For this review, take the finished solid that the model builds, in its own axes (mm). A direction names the side the tool comes from. Coordinates: 2 decimals unless noted, no trailing zeros. Write each loop counter-clockwise with the first axis right and the second up, starting at its lowest first coordinate (ties: lowest second). Pieces come first, ordered by that corner, then holes. Notation, with made-up numbers: (-18, 26) -> (35, 26) arc R21 ccw to (35, 50) -> close; hole circle Ø10 at (-14.5, 58.25). An arc over 180 degrees is marked (long way). One line per item, written item: value. Start each with the question number.
1) Machinability: for faces 1 (the flat face through (16, -6.528, 2)), 2 (the flat face through (124.565, 17.321, 1.478)), 3 (the flat face through (-38.1, -18, 2)), which of the approach directions +Z, -Z, +X, -X, +Y, -Y give a long, thin tool a straight path to every point of the face, cutting with its end or side? Answer none if there is none.
2) Add section D-D (z = 2.2). State how many separate pieces and enclosed holes the cut face has, and give its area (3 significant figures).
3) For probe 1 along Y at (x, z) = (76.2, 1.85); probe 2 along Y at (x, z) = (104.5, 2.55); probe 3 along Y at (x, z) = (127, 1.6), list the stretches that pass through material, from the lowest coordinate up. Write a range as from..to.
4) For pin 1 Ø4 at (x, y) = (76.2, 41.07) entering from -Z; pin 2 Ø0.9 at (y, z) = (-17, 1) entering from +X; pin 3 Ø0.9 at (y, z) = (-17.5, 2) entering from -X; pin 4 Ø0.9 at (x, z) = (30, 1) entering from -Y, all flat-tipped, find the tip position at first contact; note any pin that passes through.
5) Add section C-C (y = 25.4). State the section outline as (x, z) points.
6) Add section A-A (x = 76.2). State the section outline as (y, z) points.
7) Mouldability with a two-part tool opening along X and no side actions: class faces 4 (the flat face through (74.696, 8.434, 1.52)), 5 (the flat face through (70.38, -7.28, 1.48)), 6 (the flat face through (23, 15, 0)) as released by +X, released by -X, zero draft, split by the parting line, or undercut.
8) Add section B-B (x = 127). State the section outline as (y, z) points, and give its area (3 significant figures).
from build123d import *

# Parameters (mm, degrees)
BASE_DEPTH              = 2.9972
JOINT_HOLES_D           = 4.3053
JOINT_HOLES_DEPTH       = 6.351016
OUTER_FILLET_R          = 6.35
SKETCH5_W               = 12.7
SKETCH5_H               = 2.9972
BASE_PLATE_SLOTS_DEPTH  = 142.562822885
UNDER_PLATE_SLOTS_DEPTH = 142.562822885
TOP_PLATE_SLOTS_DEPTH   = 142.562822885
INNER_HOLE_DEPTH        = 142.562822885
INNER_FILLET_R          = 3.175


with BuildPart() as part:
    # Sketch2 → Base (new body)
    with BuildSketch(Plane.XY):
        with BuildLine():
            Line((-44.45, -19.05), (44.45, -19.05))
            Line((44.45, -19.05), (129.624951321, 19.617947547))
            ThreePointArc((129.624951321, 19.617947547), (133.337217148, 25.802714314), (128.871921697, 31.467817496))
            Line((128.871921697, 31.467817496), (78.071921697, 47.139617496))
            ThreePointArc((78.071921697, 47.139617496), (75.950116907, 47.416881437), (73.856688269, 46.973612445))
            Line((73.856688269, 46.973612445), (-44.45, 0))
            Line((-44.45, 0), (-44.45, -19.05))
        make_face()
    extrude(amount=BASE_DEPTH)

    # Joint holes
    with Locations(Plane.XY.offset(2.9972)):
        with Locations((76.2, 41.0718), (127, 25.4)):
            Hole(JOINT_HOLES_D / 2, depth=JOINT_HOLES_DEPTH)

    # Outer fillet
    outer_fillet_edges = [part.edges().sort_by_distance(p)[0] for p in [
        (-44.45, 0, 1.4986),
        (44.45, -19.05, 1.4986),
        (-44.45, -19.05, 1.4986),
    ]]
    fillet(outer_fillet_edges, radius=OUTER_FILLET_R)

    # Sketch5 → Base plate slots (cut, through all)
    with BuildSketch(Plane.XY.offset(2.9972)):
        with Locations((-31.75, -17.5514)):
            Rectangle(SKETCH5_W, SKETCH5_H)
        with Locations((31.75, -17.5514)):
            Rectangle(SKETCH5_W, SKETCH5_H)
    extrude(amount=-BASE_PLATE_SLOTS_DEPTH, mode=Mode.SUBTRACT)

    # Sketch6 → Under plate slots (cut, through all)
    with BuildSketch(Plane.XY.offset(2.9972)):
        Polygon((50.260345678, -16.412204047), (49.021368655, -13.683075289), (60.58547356, -8.433172648), (61.824450584, -11.162301405), align=None)
        Polygon((79.170607941, -3.287447443), (77.931630918, -0.558318686), (89.495735823, 4.691583955), (90.734712847, 1.962455198), align=None)
        Polygon((108.080870204, 9.83730916), (106.841893181, 12.566437917), (118.405998086, 17.816340558), (119.644975109, 15.087211801), align=None)
    extrude(amount=-UNDER_PLATE_SLOTS_DEPTH, mode=Mode.SUBTRACT)

    # Sketch7 → Top plate slots (cut, through all)
    with BuildSketch(Plane.XY.offset(2.9972)):
        Polygon((-37.492405509, 2.762509474), (-36.386362372, -0.023146), (-24.582737483, 4.663477462), (-25.68878062, 7.449132936), align=None)
        Polygon((3.820281603, 19.165691592), (4.92632474, 16.380036118), (16.729949629, 21.06665958), (15.623906492, 23.852315054), align=None)
        Polygon((45.132968715, 35.56887371), (46.239011852, 32.783218236), (58.042636741, 37.469841698), (56.936593604, 40.255497172), align=None)
    extrude(amount=-TOP_PLATE_SLOTS_DEPTH, mode=Mode.SUBTRACT)

    # Sketch8 → Inner hole (cut, through all)
    with BuildSketch(Plane.XY.offset(2.9972)):
        Polygon((-26.957611693, -6.5278), (80.903097736, 36.298241679), (113.752323838, 26.164255426), (41.740634412, -6.5278), align=None)
    extrude(amount=-INNER_HOLE_DEPTH, mode=Mode.SUBTRACT)

    # Inner fillet
    inner_fillet_edges = [part.edges().sort_by_distance(p)[0] for p in [
        (41.740634412, -6.5278, 1.4986),
        (-26.957611693, -6.5278, 1.4986),
        (80.903097736, 36.298241679, 1.4986),
        (113.752323838, 26.164255426, 1.4986),
    ]]
    fillet(inner_fillet_edges, radius=INNER_FILLET_R)


solid = part.part
Numbers:
1. face 1: +Z, -Z
1. face 2: +Z, -Z, +X, -Y
1. face 3: +Z, -Z, -Y
2. separate pieces: 1
2. enclosed holes: 3
2. area: 4,030 mm²
3. probe 1: -4.64..9.12, 34.43..38.92, 43.22..47.42
3. probe 2: 8.21..21.96, 29.02..38.99
3. probe 3: 18.43..23.25, 27.55..32.05
4. pin 1: through
4. pin 2: x = 49.96
4. pin 3: x = -42.73
4. pin 4: y = -16.05
5. outline: (19.52, 0) -> (53.46, 0) -> (53.46, 3) -> (19.52, 3) -> close; (107.99, 0) -> (124.85, 0) -> (124.85, 3) -> (107.99, 3) -> close; (129.15, 0) -> (133.35, 0) -> (133.35, 3) -> (129.15, 3) -> close
6. outline: (-4.64, 0) -> (9.12, 0) -> (9.12, 3) -> (-4.64, 3) -> close; (34.43, 0) -> (38.92, 0) -> (38.92, 3) -> (34.43, 3) -> close; (43.22, 0) -> (47.42, 0) -> (47.42, 3) -> (43.22, 3) -> close
7. face 4: undercut
7. face 5: released by +X
7. face 6: zero draft
8. outline: (18.43, 0) -> (23.25, 0) -> (23.25, 3) -> (18.43, 3) -> close; (27.55, 0) -> (32.05, 0) -> (32.05, 3) -> (27.55, 3) -> close
8. area: 27.9 mm²
